The model under review builds one solid part; all positions refer to its coordinate system, in mm. A direction names the side the tool comes from. Round coordinates to 2 decimals unless told otherwise and drop trailing zeros. Loops run counter-clockwise (first coordinate to the right, second up) from the corner with the lowest first, then second, coordinate; pieces in that order, holes last. Notation, with made-up numbers: M 50.25,3.5 L 98.25,3.5 A23 cw 98.25,32.5 Z; hole C 17,23.25 d3. An arc over 180 degrees is marked long. Use a Markdown table: item, result. Add a question column.
```python
from build123d import *

# Parameters (mm, degrees)
SKETCH1_W           = 317.5
SKETCH1_H           = 152.4
SKETCH1_R           = 3.175
BOSS_EXTRUDE1_DEPTH = 12.7
FILLET1_R           = 3.175


with BuildPart() as part:
    # Sketch1 → Boss-Extrude1 (new body)
    with BuildSketch(Plane(origin=(0, 0, 0), x_dir=(1, 0, 0), z_dir=(0, 1, 0))):
        with Locations((158.75, 76.2)):
            Rectangle(SKETCH1_W, SKETCH1_H)
        with Locations(Location((12.7, 25.4, 0), (0, 0, 270))):
            Circle(SKETCH1_R, mode=Mode.SUBTRACT)
        with Locations(Location((12.7, 139.7, 0), (0, 0, 270))):
            Circle(SKETCH1_R, mode=Mode.SUBTRACT)
        with Locations(Location((304.8, 139.7, 0), (0, 0, 270))):
            Circle(SKETCH1_R, mode=Mode.SUBTRACT)
        with Locations(Location((304.8, 25.4, 0), (0, 0, 270))):
            Circle(SKETCH1_R, mode=Mode.SUBTRACT)
        with Locations(Location((38.1, 25.4, 0), (0, 0, 270))):
            Circle(SKETCH1_R, mode=Mode.SUBTRACT)
        with Locations(Location((137.16, 25.4, 0), (0, 0, 270))):
            Circle(SKETCH1_R, mode=Mode.SUBTRACT)
        with Locations(Location((180.34, 25.4, 0), (0, 0, 90))):
            Circle(SKETCH1_R, mode=Mode.SUBTRACT)
        with Locations(Location((279.4, 25.4, 0), (0, 0, 90))):
            Circle(SKETCH1_R, mode=Mode.SUBTRACT)
        with BuildLine():
            Line((57.15, 38.1), (118.11, 38.1))
            ThreePointArc((118.11, 38.1), (130.81, 25.4), (118.11, 12.7))
            Line((118.11, 12.7), (57.15, 12.7))
            ThreePointArc((57.15, 12.7), (44.45, 25.4), (57.15, 38.1))
        make_face(mode=Mode.SUBTRACT)
        with BuildLine():
            Line((260.35, 38.1), (199.39, 38.1))
            ThreePointArc((199.39, 38.1), (186.69, 25.4), (199.39, 12.7))
            Line((199.39, 12.7), (260.35, 12.7))
            ThreePointArc((260.35, 12.7), (273.05, 25.4), (260.35, 38.1))
        make_face(mode=Mode.SUBTRACT)
    extrude(amount=BOSS_EXTRUDE1_DEPTH)

    # Fillet1
    fillet1_edges = [part.edges().sort_by_distance(p)[0] for p in [
        (0, 6.35, -152.4),
        (317.5, 6.35, -152.4),
        (317.5, 6.35, 0),
        (0, 6.35, 0),
    ]]
    fillet(fillet1_edges, radius=FILLET1_R)


solid = part.part
```
(1) To check wall thickness, follow probe 1 along Z at (x, y) = (304.8, 8) (3 decimals); probe 2 along X at (y, z) = (7, -139.7) (3 decimals); probe 3 along Z at (x, y) = (180.34, 5.25) (3 decimals). State the ranges of each line that lie inside material, in increasing order.
(2) Insertion check: pin 1 Ø4 at (x, z) = (137.16, -25.4) entering from +Y. The pin has a flat end and moves straight along its axis. Give the tip position at first contact, or say it passes through.
(3) Consider section A-A, the plane x = 114.5. Give the boundary of the cut face in (y, z), then the cut area to 3 significant figures.
(4) For faces 5 (the face through (157, 12.7, -77)), 6 (the face through (87, 6, -38.1)), list the 3-axis set-ups (+Z, -Z, +X, -X, +Y, -Y) from which the entire face can be reached by the end or side of a thin tool; tool diameter is ignored.
(5) Consider section B-B, the plane y = 3. Give the number of separate pieces and of enclosed holes in the cut face, then the cut area to 3 significant figures.
(6) Consider section D-D, the plane x = 304.8. Give the boundary of the cut face in (y, z) (3 decimals).
(7) Draft analysis for pull direction X (two halves, no side actions). For faces 1 (the face through (186.693, 6.261, -25.679)), 2 (the face through (0, 6, -75)), 3 (the face through (273.047, 6.261, -25.121)), 4 (the face through (317.5, 6, -75)), state which applies: released by +X, released by -X, zero draft, split by the parting line, or undercut.
(8) Consider section C-C, the plane z = -139.7. Give the boundary of the cut face in (x, y) (3 decimals).
Found:
| question | item | result |
|---|---|---|
| 1 | probe 1 | z = -152.4 to -142.875, -136.525 to -28.575, -22.225 to 0 |
| 1 | probe 2 | x = 0 to 9.525, 15.875 to 301.625, 307.975 to 317.5 |
| 1 | probe 3 | z = -152.4 to -28.575, -22.225 to 0 |
| 2 | pin 1 | passes through |
| 3 | outline | M 0,-152.4 L 12.7,-152.4 L 12.7,-38.1 L 0,-38.1 Z; M 0,-12.7 L 12.7,-12.7 L 12.7,0 L 0,0 Z |
| 3 | area | 1,610 mm^2 |
| 4 | face 5 | +Z, -Z, +X, -X, +Y |
| 4 | face 6 | +Y, -Y |
| 5 | separate pieces | 1 |
| 5 | enclosed holes | 10 |
| 5 | area | 44,000 mm^2 |
| 6 | outline | M 0,-152.4 L 12.7,-152.4 L 12.7,-142.875 L 0,-142.875 Z; M 0,-136.525 L 12.7,-136.525 L 12.7,-28.575 L 0,-28.575 Z; M 0,-22.225 L 12.7,-22.225 L 12.7,0 L 0,0 Z |
| 7 | face 1 | undercut |
| 7 | face 2 | released by -X |
| 7 | face 3 | undercut |
| 7 | face 4 | released by +X |
| 8 | outline | M 0,0 L 9.525,0 L 9.525,12.7 L 0,12.7 Z; M 15.875,0 L 301.625,0 L 301.625,12.7 L 15.875,12.7 Z; M 307.975,0 L 317.5,0 L 317.5,12.7 L 307.975,12.7 Z |
